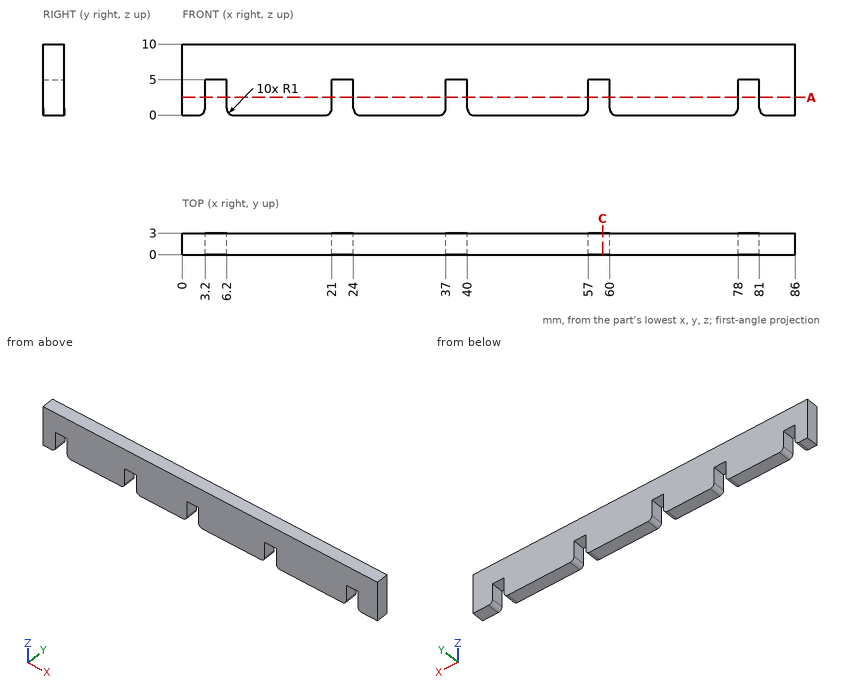
Study the drawing (mm; zero at the part's minimum x, y, z) and answer. Coordinates: 2 decimals unless noted, no trailing zeros. Write each loop counter-clockwise with the first axis right and the second up, starting at its lowest first coordinate (ties: lowest second). Pieces come first, ordered by that corner, then holes. Notation, with made-up numbers: M -9,-6 L 14,-6 A27 cw 14,26 Z; hole C 41,-24.75 d8. An arc over 180 degrees is marked long. Use one line per item in the form item = value.
Item 1: Find section A-A, the plane z = 2.5. Give the vertices of the cut face in (x, y), plus the area to 3 significant figures.
Model answer:
outline = M 0,0 L 3.2,0 L 3.2,3 L 0,3 Z; M 6.2,0 L 21,0 L 21,3 L 6.2,3 Z; M 24,0 L 37,0 L 37,3 L 24,3 Z; M 40,0 L 57,0 L 57,3 L 40,3 Z; M 60,0 L 78,0 L 78,3 L 60,3 Z; M 81,0 L 86,0 L 86,3 L 81,3 Z
area = 213 mm2
Item 2: Find section C-C, the plane x = 59. Give the vertices of the cut face in (y, z), plus the area to 3 significant figures.
Model answer:
outline = M 0,5 L 3,5 L 3,10 L 0,10 Z
area = 15.0 mm2
Item 3: Given P1, Ø0.9, axis at x = 38.5, y = 1, coming from the -Z side, flat-ended and moving along its own axis, determine where the tip first touches the part or whether it passes through.
Model answer:
P1 = 5
Item 4: Find the intervals of material crossed by probe 1 along X at (y, z) = (1.9, 2); probe 2 along Z at (x, y) = (59, 1.8), in increasing order.
Model answer:
probe_1 = 0 to 3.2, 6.2 to 21, 24 to 37, 40 to 57, 60 to 78, 81 to 86
probe_2 = 5 to 10
